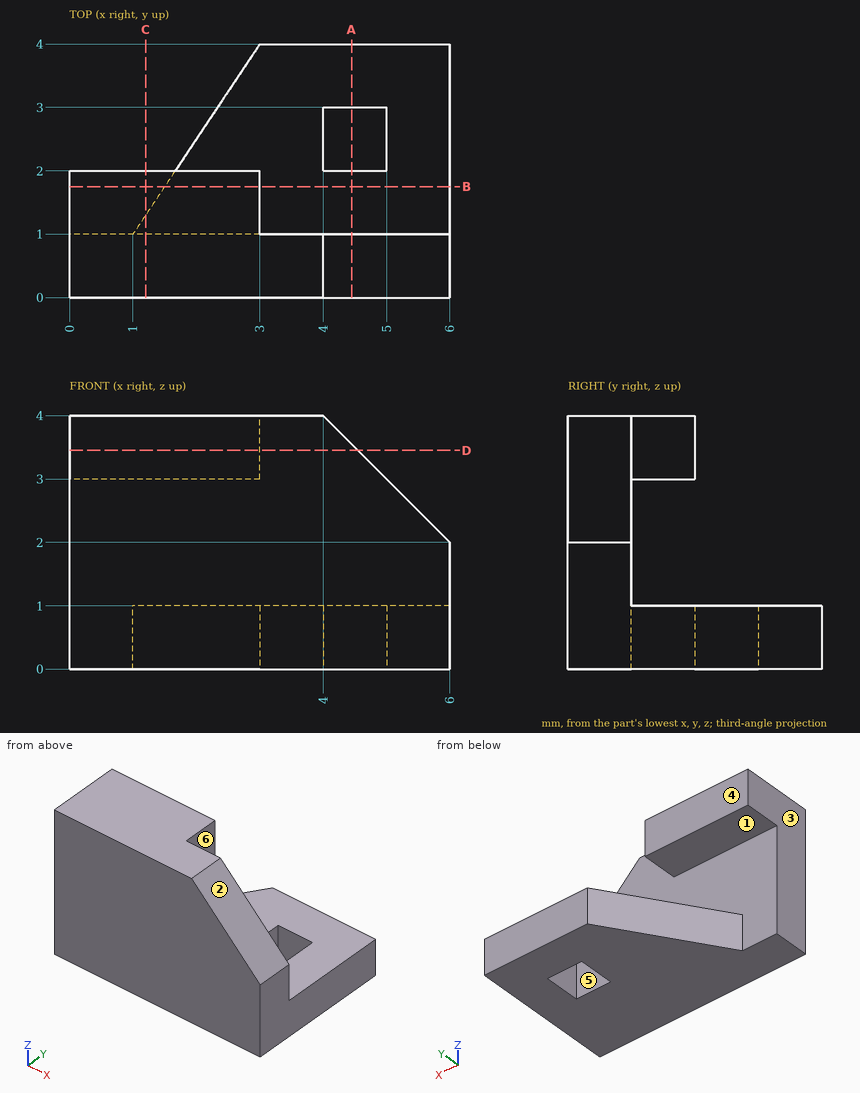
The figure shows three views and two pictorial views of one solid part (mm, origin at its lowest corner). Answer the questions. A direction names the side the tool comes from. Coordinates: 2 decimals unless noted, no trailing zeros. Loops run counter-clockwise (first coordinate to the right, second up) from the corner with the lowest first, then second, coordinate; pieces in that order, holes last. Notation, with made-up numbers: (78, 47.25) -> (115, 47.25) arc R4 cw to (115, 53.25) -> close; hole circle Ø10 at (56.25, -5.75). An arc over 180 degrees is marked (long way). Return JSON: item names as keys, results as strings. Group by question number.
(1) Find the intervals of material crossed by probe 1 along Z at (x, y) = (2.65, 1.25); probe 2 along Y at (x, z) = (4.3, 0.2); probe 3 along Z at (x, y) = (5.35, 1.7), in increasing order. Write a range as from..to.
(2) Given pin 1 Ø2 at (x, z) = (2.5, 3.5) entering from +Y, flat-ended and moving along its own axis, determine where the tip first touches the part or whether it passes through.
(3) A cutting plane is placed at A-A on x = 4.45. Write down the section's boundary in (y, z).
(4) Which of the six approach directions +Z, -Z, +X, -X, +Y, -Y give full straight-line access (tool end or side, diameter ignored) to the marked faces 4, 5 and 6?
(5) A cutting plane is placed at B-B on y = 1.75. Write down the section's boundary in (x, z), and give its area (3 significant figures).
(6) Determine the mould class of the marked faces 1, 2 and 3 for opening direction Z: released by +Z, released by -Z, zero draft, split by the parting line, or undercut.
(7) A cutting plane is placed at C-C on x = 1.2. Write down the section's boundary in (y, z).
(8) A cutting plane is placed at D-D on z = 3.45. Write down the section's boundary in (x, y).
The answers:
{
 "1": {"probe 1": "z = 0..1, 3..4", "probe 2": "y = 0..2, 3..4", "probe 3": "z = 0..1"},
 "2": {"pin 1": "stops at y = 2"},
 "3": {"outline": "(0, 0) -> (2, 0) -> (2, 1) -> (1, 1) -> (1, 3.55) -> (0, 3.55) -> close; (3, 0) -> (4, 0) -> (4, 1) -> (3, 1) -> close"},
 "4": {"face 4": "+Z, +X, -X, +Y", "face 5": "+Z, -Z", "face 6": "+Z, +X, +Y"},
 "5": {"outline": "(0, 3) -> (3, 3) -> (3, 4) -> (0, 4) -> close; (1.5, 0) -> (6, 0) -> (6, 1) -> (1.5, 1) -> close", "area": "7.50 mm^2"},
 "6": {"face 1": "undercut", "face 2": "released by +Z", "face 3": "zero draft"},
 "7": {"outline": "(0, 0) -> (1.3, 0) -> (1.3, 1) -> (1, 1) -> (1, 3) -> (2, 3) -> (2, 4) -> (0, 4) -> close"},
 "8": {"outline": "(0, 0) -> (4.55, 0) -> (4.55, 1) -> (3, 1) -> (3, 2) -> (0, 2) -> close"}
}
